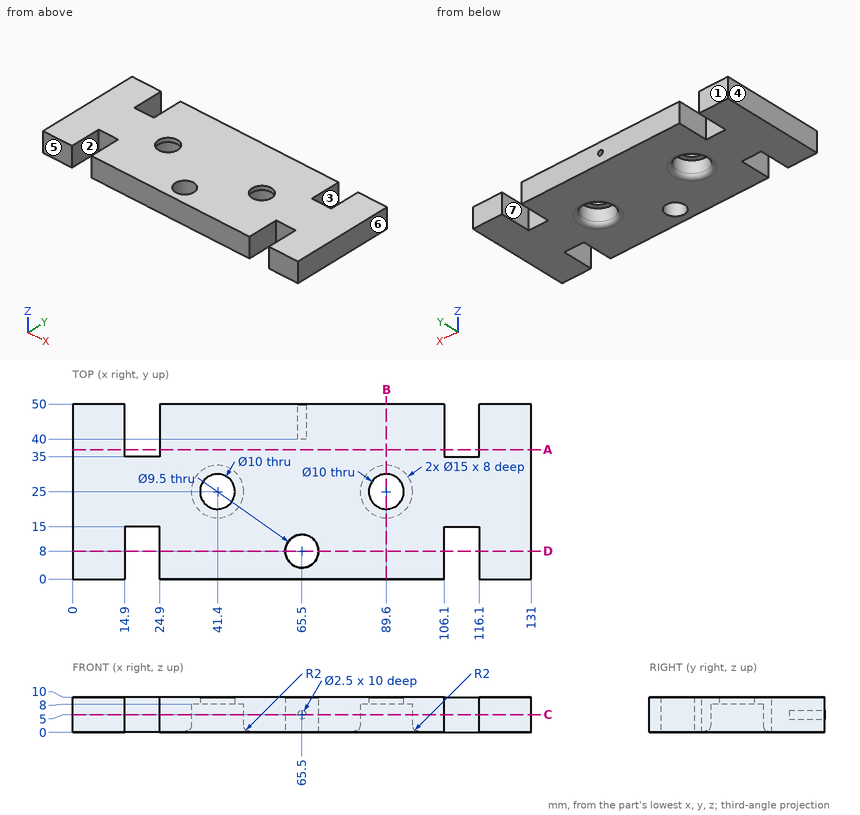
Here's the drawing with two shaded views (mm, measured from the low corner). I have some questions. A direction names the side the tool comes from. Give positions to 0.01 mm unless a question says otherwise; leave off trailing zeros. Loops run counter-clockwise (first coordinate to the right, second up) from the corner with the lowest first, then second, coordinate; pieces in that order, holes last. Notation, with made-up numbers: (-16, 52) - (21, 52) arc R23 ccw to (21, 73) - close; hole circle Ø5 at (66, 47.25). An arc over 180 degrees is marked (long way). One line per item, written item: value.
(1) I need wall thicknesses on line 1 along X through (y, z) = (3, 3); line 2 along Y through (x, z) = (41.4, 9.05); line 3 along Z through (x, y) = (65.5, 45.75). Which ranges of each line are inside material? Lowest first, please.
Verdict:
line 1: 0 to 14.9, 24.9 to 106.1, 116.1 to 131
line 2: 0 to 20, 30 to 50
line 3: 0 to 3.75, 6.25 to 10
(2) I'm going to push flat-ended pins straight in: pin 1 (3 mm diameter, centred on x = 19, z = 4.5, fed in from +Y); pin 2 (5 mm diameter, centred on x = 20.5, z = 3.5, fed in from -Y); pin 3 (17 mm diameter, centred on x = 41.4, y = 25, fed in from -Z). Where does each tip first touch, or does it pass through?
Verdict:
pin 1: y = 35
pin 2: y = 15
pin 3: z = 0.27
(3) If we section it at B-B, the plane x = 89.6: List the corners of the cut face in (y, z) for me.
Verdict:
outline: (0, 0) - (15.5, 0) arc R2 ccw to (17.5, 2) - (17.5, 8) - (20, 8) - (20, 10) - (0, 10) - close; (30, 8) - (32.5, 8) - (32.5, 2) arc R2 ccw to (34.5, 0) - (50, 0) - (50, 10) - (30, 10) - close
(4) If we mould it in two halves opening along X, with no side actions, what happens to the marked faces 4, 5, 6 and 7? For each: released by +X, released by -X, zero draft, split by the parting line, or undercut.
Verdict:
face 4: released by -X
face 5: zero draft
face 6: released by +X
face 7: undercut
(5) If we section it at C-C, the plane z = 5: List the corners of the cut face in (x, y) for me, plus the area to 3 significant figures.
Verdict:
outline: (0, 0) - (14.9, 0) - (14.9, 15) - (24.9, 15) - (24.9, 0) - (106.1, 0) - (106.1, 15) - (116.1, 15) - (116.1, 0) - (131, 0) - (131, 50) - (116.1, 50) - (116.1, 35) - (106.1, 35) - (106.1, 50) - (66.75, 50) - (66.75, 40) - (64.25, 40) - (64.25, 50) - (24.9, 50) - (24.9, 35) - (14.9, 35) - (14.9, 50) - (0, 50) - close; hole circle Ø15 at (41.4, 25); hole circle Ø9.5 at (65.5, 8); hole circle Ø15 at (89.6, 25)
area: 5,500 mm^2
(6) If we section it at D-D, the plane y = 8: List the corners of the cut face in (x, z) for me.
Verdict:
outline: (0, 0) - (14.9, 0) - (14.9, 10) - (0, 10) - close; (24.9, 0) - (60.75, 0) - (60.75, 10) - (24.9, 10) - close; (70.25, 0) - (106.1, 0) - (106.1, 10) - (70.25, 10) - close; (116.1, 0) - (131, 0) - (131, 10) - (116.1, 10) - close
(7) On a 3-axis mill with a long thin cutter (end or side, diameter ignored), from which of +Z, -Z, +X, -X, +Y, -Y can I reach the whole of each face in a straight line? I mean the marked faces 1, 2 and 3. Say none if no direction works.
Verdict:
face 1: +Z, -Z, +X, -X, +Y
face 2: +Z, -Z, -Y
face 3: +Z, -Z, +Y
(8) If we section it at A-A, the plane y = 37: List the corners of the cut face in (x, z) for me, plus the area to 3 significant figures.
Verdict:
outline: (0, 0) - (14.9, 0) - (14.9, 10) - (0, 10) - close; (24.9, 0) - (106.1, 0) - (106.1, 10) - (24.9, 10) - close; (116.1, 0) - (131, 0) - (131, 10) - (116.1, 10) - close
area: 1,110 mm^2
